```python
from build123d import *

# Parameters (mm, degrees)
CROQUIS1_W              = 200
CROQUIS1_H              = 150
SALIENTE_EXTRUIR1_DEPTH = 3
CROQUIS2_W              = 3
CROQUIS2_H              = 150
SALIENTE_EXTRUIR2_DEPTH = 30
SALIENTE_EXTRUIR4_DEPTH = 5
CROQUIS6_W              = 200
CROQUIS6_H              = 33
SALIENTE_EXTRUIR5_DEPTH = 5
CHAFL_N1_SIZE           = 10
CHAFL_N2_SIZE           = 10
CROQUIS7_R              = 1.5
CORTAR_EXTRUIR2_DEPTH   = 10
CROQUIS8_W              = 48
CROQUIS8_H              = 30
CORTAR_EXTRUIR3_DEPTH   = 200
SALIENTE_EXTRUIR6_DEPTH = 200


with BuildPart() as part:
    # Croquis1 → Saliente-Extruir1 (new body)
    with BuildSketch(Plane(origin=(0, 0, 0), x_dir=(1, 0, 0), z_dir=(0, 1, 0))):
        with Locations((100, 75)):
            Rectangle(CROQUIS1_W, CROQUIS1_H)
    extrude(amount=SALIENTE_EXTRUIR1_DEPTH)

    # Croquis2 → Saliente-Extruir2 (add)
    with BuildSketch(Plane(origin=(0, 3, 0), x_dir=(1, 0, 0), z_dir=(0, 1, 0))):
        with Locations((1.5, 75)):
            Rectangle(CROQUIS2_W, CROQUIS2_H)
        with Locations((198.5, 75)):
            Rectangle(CROQUIS2_W, CROQUIS2_H)
    extrude(amount=SALIENTE_EXTRUIR2_DEPTH)

    # Croquis5 → Saliente-Extruir4 (add)
    with BuildSketch(Plane.XY):
        Polygon((0, 33), (3, 33), (200, 33), (200, 0), (0, 0), align=None)
    extrude(amount=SALIENTE_EXTRUIR4_DEPTH)

    # Croquis6 → Saliente-Extruir5 (add)
    with BuildSketch(Plane(origin=(0, 0, -150), x_dir=(-1, 0, 0), z_dir=(0, 0, -1))):
        with Locations((-100, 16.5)):
            Rectangle(CROQUIS6_W, CROQUIS6_H)
    extrude(amount=SALIENTE_EXTRUIR5_DEPTH)

    # Chaflán1
    chafl_n1_edges = [part.edges().sort_by_distance(p)[0] for p in [
        (100, 0, 5),
        (100, 0, -155),
    ]]
    chamfer(chafl_n1_edges, length=CHAFL_N1_SIZE)

    # Chaflán2
    chafl_n2_edges = [part.edges().sort_by_distance(p)[0] for p in [
        (100, 3, 0),
        (100, 3, -150),
    ]]
    chamfer(chafl_n2_edges, length=CHAFL_N2_SIZE)

    # Croquis7 → Cortar-Extruir2 (cut)
    with BuildSketch(Plane(origin=(0, 3, 0), x_dir=(1, 0, 0), z_dir=(0, 1, 0))):
        with Locations(Location((189, 30, 0), (0, 0, 270))):
            Circle(CROQUIS7_R)
        with Locations(Location((177, 30, 0), (0, 0, 270))):
            Circle(CROQUIS7_R)
        with Locations(Location((189, 54, 0), (0, 0, 270))):
            Circle(CROQUIS7_R)
        with Locations(Location((177, 54, 0), (0, 0, 270))):
            Circle(CROQUIS7_R)
        with Locations(Location((23, 30, 0), (0, 0, 270))):
            Circle(CROQUIS7_R)
        with Locations(Location((11, 30, 0), (0, 0, 270))):
            Circle(CROQUIS7_R)
        with Locations(Location((23, 54, 0), (0, 0, 270))):
            Circle(CROQUIS7_R)
        with Locations(Location((11, 54, 0), (0, 0, 270))):
            Circle(CROQUIS7_R)
    extrude(amount=-CORTAR_EXTRUIR2_DEPTH, mode=Mode.SUBTRACT)

    # Croquis8 → Cortar-Extruir3 (cut)
    with BuildSketch(Plane(origin=(200, 0, 0), x_dir=(0, 0, -1), z_dir=(1, 0, 0))):
        with Locations((38.75, 18)):
            Rectangle(CROQUIS8_W, CROQUIS8_H)
    extrude(amount=-CORTAR_EXTRUIR3_DEPTH, mode=Mode.SUBTRACT)

    # Croquis9 → Saliente-Extruir6 (add)
    with BuildSketch(Plane(origin=(200, 0, 0), x_dir=(0, 0, -1), z_dir=(1, 0, 0))):
        Polygon((155, 10), (160.560253642, 15.560253642), (160, 33), (155, 33), align=None)
    extrude(amount=-SALIENTE_EXTRUIR6_DEPTH)


solid = part.part
```
The model under review builds one solid part; all positions refer to its coordinate system, in mm. A direction names the side the tool comes from. Round coordinates to 2 decimals unless told otherwise and drop trailing zeros. Loops run counter-clockwise (first coordinate to the right, second up) from the corner with the lowest first, then second, coordinate; pieces in that order, holes last. Notation, with made-up numbers: (23, 12.5) -> (31, 12.5) arc R29 ccw to (31, 42.5) -> close; hole circle Ø10 at (-35.5, -23.75). An arc over 180 degrees is marked (long way). Answer in a Markdown table with one row per item.
1) Wall thickness on line 1 along X through (y, z) = (1, -30); line 2 along Z through (x, y) = (189, 1.7); line 3 along X through (y, z) = (21.5, -14): over which ranges is each line inside the solid? List them lowest first.
Taken from the geometry:
| item | result |
|---|---|
| line 1 | x = 0 to 9.5, 12.5 to 21.5, 24.5 to 175.5, 178.5 to 187.5, 190.5 to 200 |
| line 2 | z = -146.7 to -55.5, -52.5 to -31.5, -28.5 to -3.3 |
| line 3 | x = 0 to 3, 197 to 200 |
2) Tool access review of faces 1 (the flat face through (100, 33, 3)), 2 (the flat face through (3, 18, -106)): name each direction out of +Z, -Z, +X, -X, +Y, -Y from which nothing blocks a thin tool from reaching the whole face with its end or side.
Taken from the geometry:
| item | result |
|---|---|
| face 1 | +Z, -Z, +X, -X, +Y |
| face 2 | +Y |
3) Consider section A-A, the plane y = 30.5. Write out the cut boundary in (x, z).
Taken from the geometry:
| item | result |
|---|---|
| outline | (0, -160.08) -> (200, -160.08) -> (200, -62.75) -> (197, -62.75) -> (197, -150) -> (3, -150) -> (3, -62.75) -> (0, -62.75) -> close; (0, -14.75) -> (3, -14.75) -> (3, 0) -> (197, 0) -> (197, -14.75) -> (200, -14.75) -> (200, 5) -> (0, 5) -> close |
4) Consider section B-B, the plane x = 154. Write out the cut boundary in (y, z), plus the area to 3 significant figures.
Taken from the geometry:
| item | result |
|---|---|
| outline | (0, -145) -> (15.56, -160.56) -> (33, -160) -> (33, -150) -> (13, -150) -> (3, -140) -> (3, -10) -> (13, 0) -> (33, 0) -> (33, 5) -> (10, 5) -> (0, -5) -> close |
| area | 888 mm² |
5) Draft analysis for pull direction X (two halves, no side actions). For faces 3 (the flat face through (197, 18, -106)), 4 (the flat face through (101, 22, 5)), 5 (the flat face through (0, 17, -95)), state which applies: pulls with the +X half, pulls with the -X half, needs draft (parallel to the pull), parting line crosses it, or undercut.
Taken from the geometry:
| item | result |
|---|---|
| face 3 | undercut |
| face 4 | needs draft |
| face 5 | pulls with the -X half |
6) Consider section C-C, the plane z = -81.5. Write out the cut boundary in (x, y).
Taken from the geometry:
| item | result |
|---|---|
| outline | (0, 0) -> (200, 0) -> (200, 33) -> (197, 33) -> (197, 3) -> (3, 3) -> (3, 33) -> (0, 33) -> close |
7) For pin 1 Ø3 at (x, y) = (29, 7) entering from -Z; pin 2 Ø1.5 at (x, y) = (167, 26.5) entering from -Z; pin 3 Ø12 at (x, z) = (32.5, -97) entering from +Y, all flat-tipped, find the tip position at first contact; note any pin that passes through.
Taken from the geometry:
| item | result |
|---|---|
| pin 1 | stops at z = -153.5 |
| pin 2 | stops at z = -160.23 |
| pin 3 | stops at y = 3 |
8) Consider section D-D, the plane z = -59. Write out the cut boundary in (x, y).
Taken from the geometry:
| item | result |
|---|---|
| outline | (0, 0) -> (200, 0) -> (200, 3) -> (0, 3) -> close |
